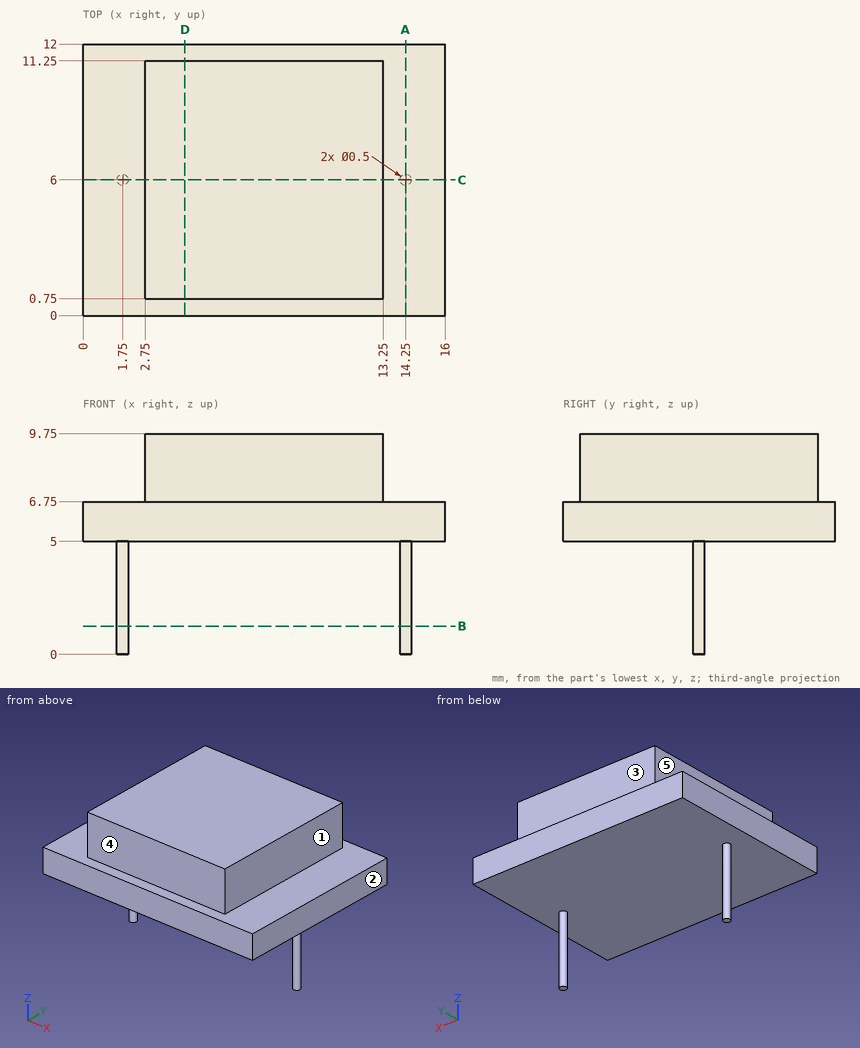
Design review of the part shown in the three views and the two pictorial views. Dimensions are in mm from the part's minimum x, y and z. A direction names the side the tool comes from. Give positions to 0.01 mm unless a question says otherwise; leave off trailing zeros. Write each loop counter-clockwise with the first axis right and the second up, starting at its lowest first coordinate (ties: lowest second). Pieces come first, ordered by that corner, then holes.
Item 1: Insertion check: P1, Ø3.5, axis at x = 8, z = 9, coming from the -Y side; P2, Ø3, axis at x = 8.5, z = 2.5, coming from the -Y side; P3, Ø6, axis at x = 9.5, y = 5.5, coming from the -Z side. Each pin has a flat end and moves straight along its axis. Give the tip position at first contact, or say it passes through.
Item 2: Take a section at C-C (y = 6). Give the boundary of the cut face in (x, z).
Item 3: Take a section at D-D (x = 4.5). Give the boundary of the cut face in (y, z), and give its area (3 significant figures).
Item 4: Take a section at A-A (x = 14.25). Give the boundary of the cut face in (y, z), and give its area (3 significant figures).
Item 5: Machinability: for the marked faces 1, 2, 3, 4 and 5, which of the approach directions +Z, -Z, +X, -X, +Y, -Y give a long, thin tool a straight path to every point of the face, cutting with its end or side? Answer none if there is none.
Item 6: Wall thickness on probe 1 along Y at (x, z) = (4.25, 9.25); probe 2 along Z at (x, y) = (4.5, 10.25); probe 3 along Z at (x, y) = (15, 6.5): over which ranges is each line inside the solid? List them lowest first.
Item 7: Take a section at B-B (z = 1.25). Give the boundary of the cut face in (x, y), and give its area (3 significant figures).
Established:
1. P1: stops at y = 0.75
1. P2: passes through
1. P3: stops at z = 5
2. outline: (0, 5) - (1.5, 5) - (1.5, 0) - (2, 0) - (2, 5) - (14, 5) - (14, 0) - (14.5, 0) - (14.5, 5) - (16, 5) - (16, 6.75) - (13.25, 6.75) - (13.25, 9.75) - (2.75, 9.75) - (2.75, 6.75) - (0, 6.75) - close
3. outline: (0, 5) - (12, 5) - (12, 6.75) - (11.25, 6.75) - (11.25, 9.75) - (0.75, 9.75) - (0.75, 6.75) - (0, 6.75) - close
3. area: 52.5 mm2
4. outline: (0, 5) - (5.75, 5) - (5.75, 0) - (6.25, 0) - (6.25, 5) - (12, 5) - (12, 6.75) - (0, 6.75) - close
4. area: 23.5 mm2
5. face 1: +Z, +X, +Y, -Y
5. face 2: +Z, -Z, +X, +Y, -Y
5. face 3: +Z, +X, -X, +Y
5. face 4: +Z, +X, -X, -Y
5. face 5: +Z, -X, +Y, -Y
6. probe 1: y = 0.75 to 11.25
6. probe 2: z = 5 to 9.75
6. probe 3: z = 5 to 6.75
7. outline: circle Ø0.5 at (1.75, 6); circle Ø0.5 at (14.25, 6)
7. area: 0.393 mm2
